Input: part model. Units: mm. Frame: model coordinates. A direction names the side the tool comes from. Coordinates: 2 decimals unless noted, no trailing zeros. Order: outer loops, then holes, each group sorted by start corner. A loop starts at its lowest first (then second) coordinate and runs counter-clockwise, first axis right, second up. Notation, with made-up numbers: (68, 66) - (94, 66) arc R14 ccw to (94, 72) - close; hole circle Ø9 at (2.5, -9.75). An arc over 180 degrees is marked (long way). Use a Markdown table: item, result. Add a question column.
from build123d import *

# Parameters (mm, degrees)
F0_W     = 30
F0_H     = 15
F1_DEPTH = 10
F2_D     = 6
F4_D     = 4
F4_DEPTH = 8
F4_TIP   = 1.2017212381
F5_W     = 16
F5_H     = 7
F6_DEPTH = 7.5


with BuildPart() as f1:
    # F0 (on Top) → F1 (new body)
    with BuildSketch(Plane.XY):
        Rectangle(F0_W, F0_H)
    extrude(amount=F1_DEPTH)

    # F2 (through all)
    with Locations(Plane(origin=(0, 0, 0), x_dir=(1, 0, 0), z_dir=(0, 0, -1))):
        with Locations((-7, 0)):
            Hole(F2_D / 2)

    # F4
    with Locations(Plane.XZ.offset(7.5)):
        with Locations((8, 5)):
            Hole(F4_D / 2, depth=F4_DEPTH)
            with Locations((0, 0, -(F4_DEPTH + F4_TIP / 2))):  # 118° drill point
                Cone(0, F4_D / 2, F4_TIP, mode=Mode.SUBTRACT)

    # F5 (on Front) → F6 (cut, symmetric)
    with BuildSketch(Plane.XZ):
        with Locations((-7, 3.5)):
            Rectangle(F5_W, F5_H)
    extrude(amount=F6_DEPTH, both=True, mode=Mode.SUBTRACT)


solid = f1.part
1) Material intervals for L1, parallel to X at y = -3.75, z = 0.5; L2, parallel to Z at x = -4, y = -5.75; L3, parallel to X at y = 0.25, z = 9, sorted ascending.
2) Contact query for a flat-ended pin moving along its axis: P1, Ø1.5, axis at x = -11, y = 0.5, coming from the -Z side. Output: stop coordinate, or through.
3) Cut plane A-A (y = 0). Return the cut outline in (x, z), and give its area (3 significant figures).
4) Cut plane B-B (x = -7). Return the cut outline in (y, z), and give its area (3 significant figures).
5) Pull-direction query (Z, two-part tool) for faces 4 (the flat face through (15, 0, 5)), 5 (the conical face through (8.187, 1.493, 5.293)), 6 (the flat face through (8, 0, 0)), 7 (the flat face through (0, 0, 10)); classes: pulls with the +Z half, pulls with the -Z half, needs draft (parallel to the pull), parting line crosses it, or undercut.
6) Cut plane C-C (z = 8.25). Return the cut outline in (x, y).
7) Cut plane D-D (y = -6.25). Return the cut outline in (x, z), and give its area (3 significant figures).
8) Reachability of faces 1 (the flat face through (3, 7.5, 6)), 2 (the flat face through (1, 0, 3)), 3 (the cylindrical face through (10, -3, 5)) from +Z, -Z, +X, -X, +Y, -Y: full face, straight path, thin tool, end or side. Return the list, or none.
Computed:
| question | item | result |
|---|---|---|
| 1 | L1 | x = 1 to 15 |
| 1 | L2 | z = 7 to 10 |
| 1 | L3 | x = -15 to -9.99, -4.01 to 15 |
| 2 | P1 | stops at z = 7 |
| 3 | outline | (-15, 7) - (-10, 7) - (-10, 10) - (-15, 10) - close; (-4, 7) - (1, 7) - (1, 0) - (15, 0) - (15, 10) - (-4, 10) - close; hole circle Ø4 at (8, 5) |
| 3 | area | 157 mm2 |
| 4 | outline | (-7.5, 7) - (-3, 7) - (-3, 10) - (-7.5, 10) - close; (3, 7) - (7.5, 7) - (7.5, 10) - (3, 10) - close |
| 4 | area | 27.0 mm2 |
| 5 | face 4 | needs draft |
| 5 | face 5 | undercut |
| 5 | face 6 | pulls with the -Z half |
| 5 | face 7 | pulls with the +Z half |
| 6 | outline | (-15, -7.5) - (15, -7.5) - (15, 7.5) - (-15, 7.5) - close; hole circle Ø6 at (-7, 0) |
| 7 | outline | (-15, 7) - (1, 7) - (1, 0) - (15, 0) - (15, 10) - (-15, 10) - close; hole circle Ø4 at (8, 5) |
| 7 | area | 175 mm2 |
| 8 | face 1 | +Z, -Z, +X, -X, +Y |
| 8 | face 2 | -Z, -X, +Y, -Y |
| 8 | face 3 | -Y |
